Geometry: final body of the model. Coordinates: model frame, mm. Face numbers are marked on the shaded views. A direction names the side the tool comes from. Give positions to 0.01 mm unless a question says otherwise; leave off trailing zeros.
Q1. Pin query (flat end, axial travel): pin 1 Ø5 at (y, z) = (13.5, 4.5) entering from -X; pin 2 Ø12 at (x, y) = (0.5, -2) entering from +Z; pin 3 Ø1 at (x, y) = (77, -64.5) entering from -Z; pin 4 Ø10 at (x, z) = (65, 10.5) entering from +Y. Return the tip coordinate at first contact, or that it passes through.
Q2. Section A-A (z = 26). State how many separate pieces and enclosed holes the cut face has, plus the area to 3 significant figures.
Q3. Line query: line 1 (Z direction, x = 48, y = -68); line 2 (Z direction, x = 20.5, y = -52); line 3 (Y direction, x = 20, z = 5). Output: solid intervals per line, ascending.
Q4. Reachability of the marked faces 1 and 2 from +Z, -Z, +X, -X, +Y, -Y: full face, straight path, thin tool, end or side. Return the list, or none.
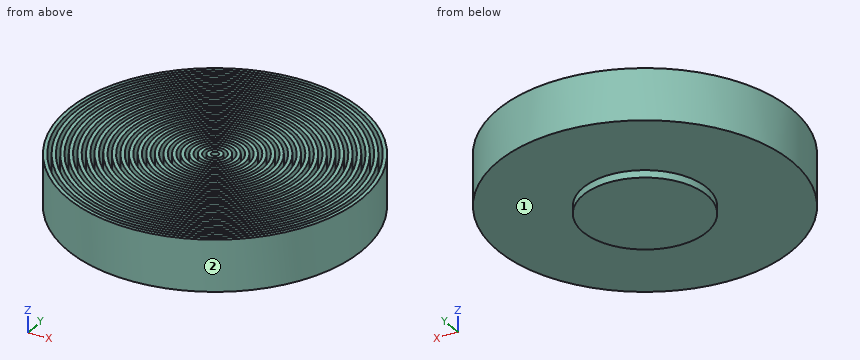
from build123d import *

# Parameters (mm, degrees)
F0_R     = 100
F1_DEPTH = 10
F2_R     = 100
F2_R_2   = 97.5
F2_R_3   = 95
F2_R_4   = 92.5
F2_R_5   = 90
F2_R_6   = 87.5
F2_R_7   = 85
F2_R_8   = 82.5
F2_R_9   = 80
F2_R_10  = 77.5
F2_R_11  = 75
F2_R_12  = 72.5
F2_R_13  = 70
F2_R_14  = 67.5
F2_R_15  = 65
F2_R_16  = 62.5
F2_R_17  = 60
F2_R_18  = 57.5
F2_R_19  = 55
F2_R_20  = 52.5
F2_R_21  = 50
F2_R_22  = 47.5
F2_R_23  = 45
F2_R_24  = 42.5
F2_R_25  = 40
F2_R_26  = 37.5
F2_R_27  = 35
F2_R_28  = 32.5
F2_R_29  = 30
F2_R_30  = 27.5
F2_R_31  = 25
F2_R_32  = 22.5
F2_R_33  = 20
F2_R_34  = 17.5
F2_R_35  = 15
F2_R_36  = 12.5
F2_R_37  = 10
F2_R_38  = 7.5
F2_R_39  = 5
F2_R_40  = 2.5
F3_DEPTH = 25
F4_R     = 41.973294
F5_DEPTH = 5


with BuildPart() as f1:
    # F0 (on Top) → F1 (new body)
    with BuildSketch(Plane.XY):
        Circle(F0_R)
    extrude(amount=F1_DEPTH)

    # F2 (on face) → F3 (join)
    with BuildSketch(Plane.XY.offset(10)):
        Circle(F2_R)
        Circle(F2_R_2, mode=Mode.SUBTRACT)
        Circle(F2_R_3)
        Circle(F2_R_4, mode=Mode.SUBTRACT)
        Circle(F2_R_5)
        Circle(F2_R_6, mode=Mode.SUBTRACT)
        Circle(F2_R_7)
        Circle(F2_R_8, mode=Mode.SUBTRACT)
        Circle(F2_R_9)
        Circle(F2_R_10, mode=Mode.SUBTRACT)
        Circle(F2_R_11)
        Circle(F2_R_12, mode=Mode.SUBTRACT)
        Circle(F2_R_13)
        Circle(F2_R_14, mode=Mode.SUBTRACT)
        Circle(F2_R_15)
        Circle(F2_R_16, mode=Mode.SUBTRACT)
        Circle(F2_R_17)
        Circle(F2_R_18, mode=Mode.SUBTRACT)
        Circle(F2_R_19)
        Circle(F2_R_20, mode=Mode.SUBTRACT)
        Circle(F2_R_21)
        Circle(F2_R_22, mode=Mode.SUBTRACT)
        Circle(F2_R_23)
        Circle(F2_R_24, mode=Mode.SUBTRACT)
        Circle(F2_R_25)
        Circle(F2_R_26, mode=Mode.SUBTRACT)
        Circle(F2_R_27)
        Circle(F2_R_28, mode=Mode.SUBTRACT)
        Circle(F2_R_29)
        Circle(F2_R_30, mode=Mode.SUBTRACT)
        Circle(F2_R_31)
        Circle(F2_R_32, mode=Mode.SUBTRACT)
        Circle(F2_R_33)
        Circle(F2_R_34, mode=Mode.SUBTRACT)
        Circle(F2_R_35)
        Circle(F2_R_36, mode=Mode.SUBTRACT)
        Circle(F2_R_37)
        Circle(F2_R_38, mode=Mode.SUBTRACT)
        Circle(F2_R_39)
        Circle(F2_R_40, mode=Mode.SUBTRACT)
    extrude(amount=F3_DEPTH)

    # F4 (on face) → F5 (join)
    with BuildSketch(Plane(origin=(0, 0, 0), x_dir=(1, 0, 0), z_dir=(0, 0, -1))):
        Circle(F4_R)
    extrude(amount=F5_DEPTH)


solid = f1.part
Computed:
1. pin 1: stops at x = -99.39
1. pin 2: stops at z = 35
1. pin 3: stops at z = 0
1. pin 4: stops at y = 80
2. separate pieces: 20
2. enclosed holes: 20
2. area: 16,100 mm2
3. line 1: z = 0 to 35
3. line 2: z = 0 to 10
3. line 3: y = -97.98 to 97.98
4. face 1: -Z
4. face 2: +Z, -Z
